Solid Edge part; units mm, degrees
sketch "Sketch1" plane through (0, 0, 0) normal (0, 0, -1) x (-1, 0, 0)
  line L0 (-30.352, 30.3553) -> (30.3477, 30.3553)
  line L1 (30.3477, 30.3553) -> (30.3477, -30.3447)
  line L2 (30.3477, -30.3447) -> (-30.352, -30.3447)
  line L3 (-30.352, -30.3447) -> (-30.352, 30.3553)
extrude "Ajout_matière_1" add sketch "Sketch1" against normal blind 81.5 and the other way blind 61.5
sketch "Sketch2" plane through (0.0021, 0.0053, 81.5) normal (0, 0, 1) x (1, 0, 0)
  line L0 (26.3749, 28.1905) -> (26.3749, -26.3875)
  line L1 (-19.6528, -26.3875) -> (26.3749, -26.3875)
extrude "Cutout1" cut sketch "Sketch2" against normal blind 48.0107 material side at (26.327, 0.9068, 81.5)
sketch "Sketch3" plane through (0.0021, 0.0053, -61.5) normal (0, 0, -1) x (0, -1, 0)
  line L0 (-25.6, 25.6001) -> (25.6, 25.6001)
  line L1 (25.6, -25.5999) -> (25.6, 25.6001)
  line L2 (-25.6, -25.5999) -> (25.6, -25.5999)
  line L3 (-25.6, -25.5999) -> (-25.6, 25.6001)
extrude "Enlèvement_matière_3" cut sketch "Sketch3" against normal blind 28
sketch "Sketch4" plane through (0.0021, -30.3447, 10) normal (0, -1, 0) x (1, 0, 0)
  circle A0 centre (0.1039, -60.1681) radius 6.75
  circle A1 centre (0, 59.948) radius 6.75
extrude "Enlèvement_matière_4" cut sketch "Sketch4" against normal blind 1.2
sketch "Sketch5" plane through (0.0021, -30.3447, 10) normal (0, -1, 0) x (1, 0, 0)
  circle A0 centre (0, 59.948) radius 3
  circle A1 centre (0.1039, -60.1681) radius 3
extrude "Cutout2" cut sketch "Sketch5" against normal up to vertex (4.75 mm away)
sketch "Sketch6" plane through (30.352, 0.0053, 10) normal (1, 0, 0) x (0, 1, 0)
  circle A0 centre (0, 59.948) radius 5.6829
  circle A1 centre (0, -60.1681) radius 5.6829
extrude "Enlèvement_matière_6" cut sketch "Sketch6" against normal blind 1.2
sketch "Sketch7" plane through (30.352, 0.0053, 10) normal (1, 0, 0) x (0, 1, 0)
  circle A0 centre (0, 59.948) radius 3
  circle A1 centre (0, -60.1681) radius 3
extrude "Cutout3" cut sketch "Sketch7" against normal up to vertex (4.75 mm away)
fillet "Congé_1" radius 2 3 edges at (-1.9853, -26.3822, 33.4893) (26.3771, 1.9865, 33.4893) (26.3771, -26.3822, 57.4946)
fillet "Congé_2" radius 2 10 edges at (30.352, 0.0053, 81.5) (28.3645, 30.3553, 81.5) (-30.3477, -28.3635, 81.5) (0.0021, -30.3447, 81.5) (-30.3477, -30.3447, 10) (30.352, -30.3447, 10) (0.0021, -30.3447, -61.5) (-30.3477, 0.0053, -61.5) (30.352, 0.0053, -61.5) (0.0021, 30.3553, -61.5)
fillet "Congé_3" radius 2 8 edges at (25.602, -25.5947, -47.5) (25.602, 0.0053, -33.5) (0.002, -25.5947, -33.5) (0.002, 25.6053, -33.5) (-25.598, 0.0053, -33.5) (-25.598, 25.6053, -47.5) (25.602, 25.6053, -47.5) (-25.598, -25.5947, -47.5)
sketch "Sketch8" plane through (0.0021, -30.3447, 10) normal (0, -1, 0) x (-1, 0, 0)
  line L0 (-12.5, -49.5) -> (12.5, -49.5)
  line L1 (12.5, -49.5) -> (12.5, -24.5)
  line L2 (12.5, -24.5) -> (-12.5, -24.5)
  line L3 (-12.5, -24.5) -> (-12.5, -49.5)
  dimension "D1" = 12.5
  dimension "D2" = 12.5
extrude "Ajout_matière_2" add sketch "Sketch8" along normal blind 8.5
sketch "Sketch9" plane through (0.0021, -34.0947, 34.5) normal (0, 0, -1) x (0, -1, 0)
  line L0 (-3.75, 14.5491) -> (-3.75, -15.4438)
  line L1 (-3.75, -15.4438) -> (1.25, -15.4438)
  line L2 (1.25, -15.4438) -> (1.25, 14.5491)
  line L3 (1.25, 14.5491) -> (-3.75, 14.5491)
  dimension "D1" = 1.25
extrude "Enlèvement_matière_8" cut sketch "Sketch9" against normal blind 15
sketch "Sketch10" plane through (30.352, 1.0053, 10) normal (1, 0, 0) x (0, -1, 0)
  line L0 (13.5, -49.5) -> (-11.5, -49.5)
  line L1 (-11.5, -49.5) -> (-11.5, -24.5)
  line L2 (-11.5, -24.5) -> (13.5, -24.5)
  line L3 (13.5, -24.5) -> (13.5, -49.5)
  dimension "D1" = 11.5
  dimension "D2" = 11.5
extrude "Ajout_matière_3" add sketch "Sketch10" along normal blind 8.5
sketch "Sketch11" plane through (34.102, 0.0053, 34.5) normal (0, 0, -1) x (1, 0, 0)
  line L0 (-3.75, 15.8991) -> (-3.75, -18.3602)
  line L1 (-3.75, -18.3602) -> (1.25, -18.3602)
  line L2 (1.25, -18.3602) -> (1.25, 15.8991)
  line L3 (1.25, 15.8991) -> (-3.75, 15.8991)
  dimension "D1" = 1.25
extrude "Enlèvement_matière_9" cut sketch "Sketch11" against normal blind 15
fillet "Congé_4" radius 1 18 edges at (38.852, 0.0053, 34.5) (38.852, -12.4947, 47) (38.852, 0.0053, 59.5) (38.852, 12.5053, 47) (35.352, 0.0053, 34.5) (12.5021, -38.8447, 47) (0.0021, -38.8447, 59.5) (0.0021, -38.8447, 34.5) (0.0021, -35.3447, 34.5) (-12.4979, -38.8447, 47) (-12.4979, -37.0947, 34.5) (12.5021, -37.0947, 34.5) (-12.4979, -34.5947, 59.5) (12.5021, -34.5947, 59.5) (34.602, -12.4947, 59.5) (37.102, -12.4947, 34.5) (34.602, 12.5053, 59.5) (37.102, 12.5053, 34.5)
The listing builds one solid part. Answer for the finished solid, in the listing's coordinates (mm). A direction names the side the tool comes from. Coordinates: 2 decimals unless noted, no trailing zeros. Loops run counter-clockwise (first coordinate to the right, second up) from the corner with the lowest first, then second, coordinate; pieces in that order, holes last. Notation, with made-up numbers: (40.5, 8) -> (77.5, 8) arc R14 ccw to (77.5, 14) -> close; hole circle Ø9 at (20.25, -23). An arc over 180 degrees is marked (long way). Answer in a Markdown table with one row per item. Add a question column.
1. Flat-ended cylindrical pins translate along their axes: P1, Ø2, axis at x = 35.5, y = 0.5, coming from the +Z side; P2, Ø1.6, axis at x = 2.5, y = -37, coming from the -Z side; P3, Ø7, axis at y = 0.01, z = 69.95, coming from the +X side; P4, Ø10, axis at x = 31.5, y = -0.5, coming from the +Z side. Find the tip coordinate at first contact, or state that the pin passes through.
2. The part is cut by section C-C, the plane x = -22. Write down the section's boundary in (y, z), then the cut area to 3 significant figures.
3. The part is cut by section B-B, the plane y = -20. Write down the section's boundary in (x, z), then the cut area to 3 significant figures.
4. Consider line 1 (X direction, y = 9.5, z = 44); line 2 (Y direction, x = -7, z = -46); line 3 (X direction, y = -23.5, z = -37). Determine where each line is inside the solid, lowest interval first. Write a range as [from, to].
5. The part is cut by section D-D, the plane z = -15.5. Write down the section's boundary in (x, y), then the cut area to 3 significant figures.
6. Determine the mould class of faces 6 (the flat face through (27, -12, 81.5)), 7 (the cylindrical face through (-0.773, -29.753, -43.476)), 8 (the flat face through (-12.498, -35, 50)) for opening direction X: +X half, -X half, draft (parallel to the pull), parting line (faces both ways), or undercut.
7. The part is cut by section A-A, the plane z = 43. Write down the section's boundary in (x, y).
8. For faces 1 (the flat face through (36, -12.495, 49)), 2 (the cylindrical face through (-0.88, -29.75, 76.64)), 3 (the flat face through (26.377, 3, 59)), 4 (the flat face through (25.602, 0, -46)), 5 (the flat face through (33, 0, 49.5)), determine the directions among +Z, -Z, +X, -X, +Y, -Y from which every point of the face is accessible in a straight line to the end or side of a thin tool.
Answer below:
| question | item | result |
|---|---|---|
| 1 | P1 | z = 59.5 |
| 1 | P2 | z = 34.5 |
| 1 | P3 | x = 29.15 |
| 1 | P4 | z = 81.5 |
| 2 | outline | (-30.34, -59.5) arc R2 ccw to (-28.34, -61.5) -> (-25.59, -61.5) -> (-25.59, -35.5) arc R2 cw to (-23.59, -33.5) -> (23.61, -33.5) arc R2 cw to (25.61, -35.5) -> (25.61, -61.5) -> (28.36, -61.5) arc R2 ccw to (30.36, -59.5) -> (30.36, 33.49) -> (-24.38, 33.49) arc R2 cw to (-26.38, 35.49) -> (-26.38, 81.5) -> (-28.34, 81.5) arc R2 ccw to (-30.34, 79.5) -> close |
| 2 | area | 4,520 mm2 |
| 3 | outline | (-30.35, -59.5) arc R2 ccw to (-28.35, -61.5) -> (-25.6, -61.5) -> (-25.6, -35.5) arc R2 cw to (-23.6, -33.5) -> (23.6, -33.5) arc R2 cw to (25.6, -35.5) -> (25.6, -61.5) -> (28.35, -61.5) arc R2 ccw to (30.35, -59.5) -> (30.35, 79.5) arc R2 ccw to (28.35, 81.5) -> (26.38, 81.5) -> (26.38, 35.49) arc R2 cw to (24.38, 33.49) -> (-30.35, 33.49) -> close |
| 3 | area | 4,520 mm2 |
| 4 | line 1 | [26.38, 30.35], [35.35, 38.85] |
| 4 | line 2 | [-30.34, -25.59], [25.61, 30.36] |
| 4 | line 3 | [-30.35, -25.6], [25.6, 30.35] |
| 5 | outline | (-30.35, -28.34) arc R2 ccw to (-28.35, -30.34) -> (28.35, -30.34) arc R2 ccw to (30.35, -28.34) -> (30.35, 30.36) -> (-30.35, 30.36) -> close |
| 5 | area | 3,680 mm2 |
| 6 | face 6 | draft |
| 6 | face 7 | undercut |
| 6 | face 8 | -X half |
| 7 | outline | (-30.35, -28.34) arc R2 ccw to (-28.35, -30.34) -> (28.35, -30.34) arc R2 ccw to (30.35, -28.34) -> (30.35, 30.36) -> (26.38, 30.36) -> (26.38, -24.38) arc R2 cw to (24.38, -26.38) -> (-30.35, -26.38) -> close; (-12.5, -37.84) arc R1 ccw to (-11.5, -38.84) -> (11.5, -38.84) arc R1 ccw to (12.5, -37.84) -> (12.5, -35.34) -> (-12.5, -35.34) -> close; (35.35, -12.49) -> (37.85, -12.49) arc R1 ccw to (38.85, -11.49) -> (38.85, 11.51) arc R1 ccw to (37.85, 12.51) -> (35.35, 12.51) -> close |
| 8 | face 1 | +Z, -Z, +X, -Y |
| 8 | face 2 | -Y |
| 8 | face 3 | +Z, -X, +Y |
| 8 | face 4 | -Z |
| 8 | face 5 | -Z, +Y, -Y |
